Verification items for the finished model (mm, model axes). Face numbers are marked on the shaded views. A direction names the side the tool comes from. Round coordinates to 2 decimals unless told otherwise and drop trailing zeros. Write each loop counter-clockwise with the first axis right and the second up, starting at its lowest first coordinate (ties: lowest second). Pieces come first, ordered by that corner, then holes. Notation, with made-up numbers: (42.25, 23) - (76.25, 23) arc R29 cw to (76.25, 46) - close; hole circle Ø3 at (51.25, 81). An arc over 180 degrees is marked (long way). Answer as a JSON object with one key per item and string values.
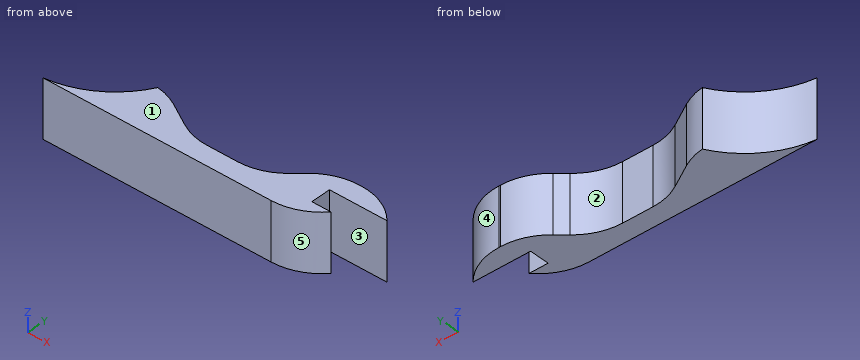
```python
from build123d import *

# Parameters (mm, degrees)
F1_DEPTH    = 7.62
F2_T1_DEPTH = 7.62
F2_T3_DEPTH = 7.62
F2_T5_DEPTH = 22.4683303368
F2_T7_DEPTH = 17.3475037725
F3_T1_DEPTH = 36.0180633142


# Not quite as in the source:
# - a fillet or chamfer that OpenCascade refuses, or shapes differently, is made with other operations: its cross-section is extruded or revolved along the edge and cut away or added


with BuildPart() as f1:
    # F0 (on Top) → F1 (new body)
    with BuildSketch(Plane.XY):
        with BuildLine():
            Line((-9.525, 0), (0, 0))
            Line((0, 0), (23.8125, 0))
            Line((23.8125, 0), (26.3525, 0))
            Line((26.3525, 0), (26.3525, 2.54))
            Line((26.3525, 2.54), (23.8125, 2.54))
            Line((23.8125, 2.54), (23.8125, 5.1562))
            Line((23.8125, 5.1562), (31.4325, 5.1562))
            Line((31.4325, 5.1562), (31.4325, 7.6962))
            Line((31.4325, 7.6962), (22.5425, 7.6962))
            Line((22.5425, 7.6962), (16.9319740389, 2.54))
            Line((16.9319740389, 2.54), (7.8691135768, 2.54))
            Line((7.8691135768, 2.54), (1.27, 6.35))
            Line((1.27, 6.35), (0, 6.35))
            ThreePointArc((0, 6.35), (-3.9738865155, 1.9920797732), (-9.525, 0))
        make_face()
    extrude(amount=F1_DEPTH)

    # F2: fillet of radius 7.62 on 4 edges, made by hand

    # F2_s2 → F2_t1 (join)
    with BuildSketch(Plane.XY):
        with BuildLine():
            ThreePointArc((13.9623079716, 2.54), (16.729273112, 3.0601194438), (19.1185079716, 4.5494740389))
            Line((19.1185079716, 4.5494740389), (16.9319740389, 2.54))
            Line((16.9319740389, 2.54), (13.9623079716, 2.54))
        make_face()
    extrude(amount=F2_T1_DEPTH)

    # F2_s4 → F2_t3 (join)
    with BuildSketch(Plane.XY):
        with BuildLine():
            ThreePointArc((9.9108864232, 2.54), (7.9386852995, 2.7996452037), (6.1008864232, 3.5608864232))
            Line((6.1008864232, 3.5608864232), (7.8691135768, 2.54))
            Line((7.8691135768, 2.54), (9.9108864232, 2.54))
        make_face()
    extrude(amount=F2_T3_DEPTH)

    # F2_s6 → F2_t5 (cut)
    with BuildSketch(Plane.XY.offset(-7.4241651684)):
        with BuildLine():
            ThreePointArc((25.5121660674, 7.6962), (22.7452009269, 7.1760805562), (20.3559660674, 5.6867259611))
            Line((20.3559660674, 5.6867259611), (22.5425, 7.6962))
            Line((22.5425, 7.6962), (25.5121660674, 7.6962))
        make_face()
    extrude(amount=F2_T5_DEPTH, mode=Mode.SUBTRACT)

    # F2_s8 → F2_t7 (cut)
    with BuildSketch(Plane.XY.offset(-4.8637518862)):
        with BuildLine():
            ThreePointArc((0, 6.35), (1.5275951478, 6.0160183482), (2.9548530765, 5.3772496228))
            Line((2.9548530765, 5.3772496228), (1.27, 6.35))
            Line((1.27, 6.35), (0, 6.35))
        make_face()
    extrude(amount=F2_T7_DEPTH, mode=Mode.SUBTRACT)

    # F3: fillet of radius 7.62 on 2 edges, made by hand

    # F3_s2 → F3_t1 (cut)
    with BuildSketch(Plane.XY.offset(-14.1990316571)):
        with BuildLine():
            ThreePointArc((25.7528873372, 7.6962), (28.8637393105, 7.0322764803), (31.4325, 5.1562))
            Line((31.4325, 5.1562), (31.4325, 7.6962))
            Line((31.4325, 7.6962), (25.7528873372, 7.6962))
        make_face()
        with BuildLine():
            ThreePointArc((26.3525, 2.54), (23.7837393105, 0.6639235197), (20.6728873372, 0))
            Line((20.6728873372, 0), (26.3525, 0))
            Line((26.3525, 0), (26.3525, 2.54))
        make_face()
    extrude(amount=F3_T1_DEPTH, mode=Mode.SUBTRACT)


solid = f1.part
```
1. Cross-section at D-D (y = 1). Record the boundary of the cut face in (x, z), plus the area to 3 significant figures.
Completed:
{"outline": "(-5.77, 0) - (24.45, 0) - (24.45, 7.62) - (-5.77, 7.62) - close", "area": "230 mm^2"}
2. Cross-section at C-C (x = 12.5). Record the boundary of the cut face in (y, z).
Completed:
{"outline": "(0, 0) - (2.54, 0) - (2.54, 7.62) - (0, 7.62) - close"}
3. Cross-section at B-B (y = 3). Record the boundary of the cut face in (x, z), plus the area to 3 significant figures.
Completed:
{"outline": "(-2.66, 0) - (7.3, 0) - (7.3, 7.62) - (-2.66, 7.62) - close; (16.57, 0) - (23.81, 0) - (23.81, 7.62) - (16.57, 7.62) - close", "area": "131 mm^2"}
4. Material ranges on probe 1 along X at (y, z) = (4.75, 3.5); probe 2 along X at (y, z) = (3.5, 3.75); probe 3 along Y at (x, z) = (10, 2), recorded low to high. Write a range as from..to.
Completed:
{"probe 1": "x = -1.03..4.04, 19.34..23.81", "probe 2": "x = -2.13..6.21, 17.66..23.81", "probe 3": "y = 0..2.54"}
5. Go/stop test with flat-tipped pins: pin 1 (2 mm diameter, centred on x = 11.5, z = 3, fed in from +Y); pin 2 (4 mm diameter, centred on x = 2.5, z = 1.5, fed in from +Y); pin 3 (2.5 mm diameter, centred on x = 27, z = 4, fed in from -Y). Record where each tip stops, or that it passes through.
Completed:
{"pin 1": "stops at y = 2.54", "pin 2": "stops at y = 6.28", "pin 3": "stops at y = 1.94"}
6. Access from +Z, -Z, +X, -X, +Y, -Y to the whole of each face (thin tool, end or side, straight path). Record for the marked faces 1 and 2.
Completed:
{"face 1": "+Z, +X, -X, +Y, -Y", "face 2": "+Z, -Z, +Y"}
7. Mould release check, pull along Y, two halves, no side actions. Record for the marked faces 3, 4 and 5: released by +Y, released by -Y, zero draft, split by the parting line, or undercut.
Completed:
{"face 3": "undercut", "face 4": "released by +Y", "face 5": "released by -Y"}
